```python
from build123d import *

# Parameters (mm, degrees)
BASE_FLANGE1_DEPTH      = 1.4
CUT_EXTRUDE1_DEPTH      = 190.741824593
CUT_EXTRUDE1_DEPTH_BACK = 190.741824593
MOTOR_HOLE_R            = 20
CUT_EXTRUDE2_DEPTH      = 190.741824593
CUT_EXTRUDE2_DEPTH_BACK = 190.741824593
SKETCH9_R               = 1.7


# Sheet-metal steps are written as plain solids
with BuildPart() as part:
    # Sketch1 → Base-Flange1 (new body)
    with BuildSketch(Plane.XY):
        Polygon((0, 0), (84.852813742, 84.852813742), (0, 169.705627485), (-84.852813742, 84.852813742), align=None)
    extrude(amount=-BASE_FLANGE1_DEPTH)

    # Motor hole → Cut-Extrude1 (cut, two sides: drawn at the far end of the back side and taken through both)
    with BuildSketch(Plane.XY.offset(-CUT_EXTRUDE1_DEPTH_BACK)):
        with Locations((0, 84.852813742)):
            Circle(MOTOR_HOLE_R)
    extrude(amount=CUT_EXTRUDE1_DEPTH + CUT_EXTRUDE1_DEPTH_BACK, mode=Mode.SUBTRACT)

    # Sketch9 → Cut-Extrude2 (cut, two sides: drawn at the far end of the back side and taken through both)
    with BuildSketch(Plane.XY.offset(-CUT_EXTRUDE2_DEPTH_BACK)):
        with Locations((-41.1, 99.852813742)):
            Circle(SKETCH9_R)
        with Locations((-25.5, 99.852813742)):
            Circle(SKETCH9_R)
        with Locations((-41.1, 69.852813742)):
            Circle(SKETCH9_R)
        with Locations((-25.5, 69.852813742)):
            Circle(SKETCH9_R)
        with Locations((25.5, 99.852813742)):
            Circle(SKETCH9_R)
        with Locations((41.1, 99.852813742)):
            Circle(SKETCH9_R)
        with Locations((25.5, 69.852813742)):
            Circle(SKETCH9_R)
        with Locations((41.1, 69.852813742)):
            Circle(SKETCH9_R)
    extrude(amount=CUT_EXTRUDE2_DEPTH + CUT_EXTRUDE2_DEPTH_BACK, mode=Mode.SUBTRACT)


solid = part.part
```
Here's how the part is built. I have some questions about the finished solid (model axes, mm). Coordinates: 2 decimals unless noted, no trailing zeros. Write each loop counter-clockwise with the first axis right and the second up, starting at its lowest first coordinate (ties: lowest second). Pieces come first, ordered by that corner, then holes. Notation, with made-up numbers: (48.5, -18) -> (88.5, -18) arc R23 ccw to (88.5, -10) -> close; hole circle Ø4 at (74, 25). An arc over 180 degrees is marked (long way). Use a Markdown table: item, result. Add a question column.
(1) Please list where these lines run through material, in increasing order: line 1 (Y direction, x = -25.5, z = -0.5); line 2 (Y direction, x = 42.5, z = -0.1); line 3 (X direction, y = 69, z = -0.9).
(2) If we section it at C-C, the plane z = -0.8: State how many separate pieces and enclosed holes the cut face has, and give its area (3 significant figures).
(3) If we section it at A-A, the plane y = 96: Write out the boundary of the cut face in (x, z).
(4) If we section it at B-B, the plane x = -2.5: Write out the boundary of the cut face in (y, z), and give its area (3 significant figures).
(5) We'd pull the mould along X, two halves only. Please class faces 1 (the cylindrical face through (-4.34, 65.33, -0.71)), 2 (the flat face through (-41.832, 127.873, -0.69)), 3 (the flat face through (-1, 105, 0)): +X half, -X half, draft (parallel to the pull), parting line (faces both ways), or undercut.
(6) If we section it at D-D, the plane y = 27: Write out the boundary of the cut face in (x, z).
(7) I'm going to push a flat-ended pin straight in: P1, Ø3, axis at x = -41.1, y = 99.85, coming from the +Z side. Where does the tip first touch, or does it pass through?
Outcome:
| question | item | result |
|---|---|---|
| 1 | line 1 | y = 25.5 to 68.15, 71.55 to 98.15, 101.55 to 144.21 |
| 1 | line 2 | y = 42.5 to 68.89, 70.82 to 98.89, 100.82 to 127.21 |
| 1 | line 3 | x = -69 to -42.57, -39.63 to -26.97, -24.03 to -12.19, 12.19 to 24.03, 26.97 to 39.63, 42.57 to 69 |
| 2 | separate pieces | 1 |
| 2 | enclosed holes | 9 |
| 2 | area | 13,100 mm^2 |
| 3 | outline | (-73.71, -1.4) -> (-16.61, -1.4) -> (-16.61, 0) -> (-73.71, 0) -> close; (16.61, -1.4) -> (73.71, -1.4) -> (73.71, 0) -> (16.61, 0) -> close |
| 4 | outline | (2.5, -1.4) -> (65.01, -1.4) -> (65.01, 0) -> (2.5, 0) -> close; (104.7, -1.4) -> (167.21, -1.4) -> (167.21, 0) -> (104.7, 0) -> close |
| 4 | area | 175 mm^2 |
| 5 | face 1 | undercut |
| 5 | face 2 | -X half |
| 5 | face 3 | draft |
| 6 | outline | (-27, -1.4) -> (27, -1.4) -> (27, 0) -> (-27, 0) -> close |
| 7 | P1 | passes through |
